Answer from the drawing. Dimensions are ordinates in mm from the lowest x, y and z of the part. Coordinates: 2 decimals unless noted, no trailing zeros. Write each loop counter-clockwise with the first axis right and the second up, starting at its lowest first coordinate (ties: lowest second). Pieces come first, ordered by that corner, then holes. Notation, with made-up numbers: (62.25, 21) - (102.25, 21) arc R22 cw to (102.25, 31) - close; hole circle Ø3 at (-13, -35.75). An arc over 180 degrees is marked (long way). Use a Markdown table: item, result.
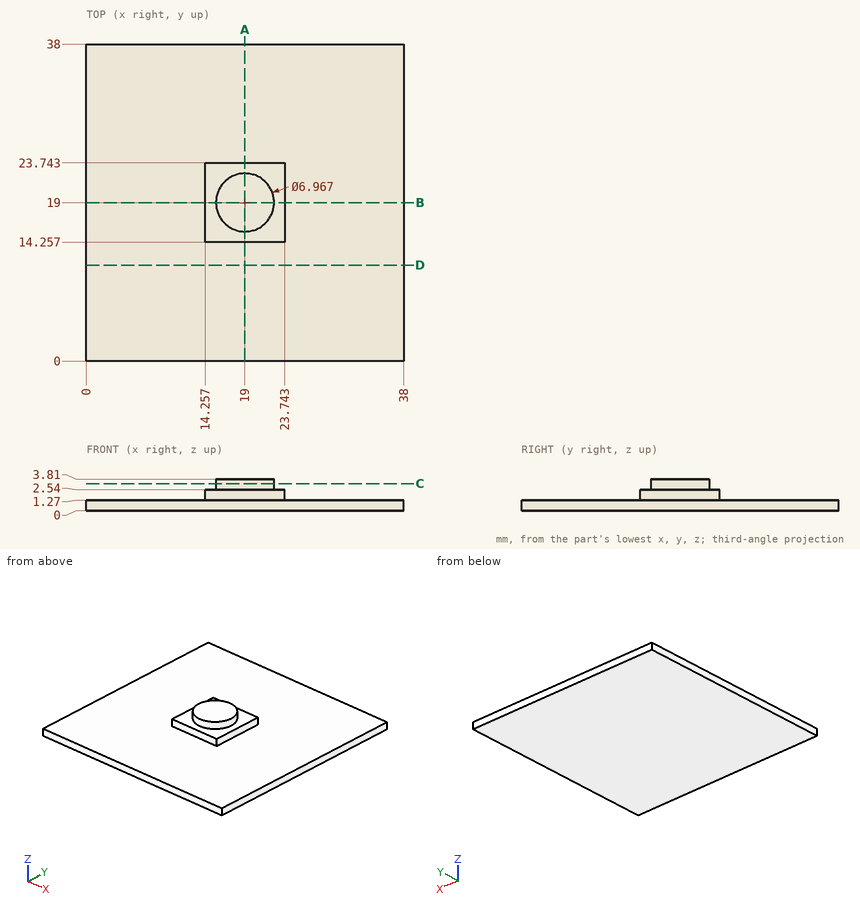
(1) A cutting plane is placed at A-A, the plane x = 19. Write down the section's boundary in (y, z).
Report:
| item | result |
|---|---|
| outline | (0, 0) - (38, 0) - (38, 1.27) - (23.74, 1.27) - (23.74, 2.54) - (22.48, 2.54) - (22.48, 3.81) - (15.52, 3.81) - (15.52, 2.54) - (14.26, 2.54) - (14.26, 1.27) - (0, 1.27) - close |
(2) Straight lines are drawn through the part: L1, parallel to Z at x = 16.5, y = 30; L2, parallel to Y at x = 22, z = 3.45; L3, parallel to Y at x = 18.5, z = 3. For each, find the intervals that lie inside material, in ascending order.
Report:
| item | result |
|---|---|
| L1 | z = 0 to 1.27 |
| L2 | y = 17.23 to 20.77 |
| L3 | y = 15.55 to 22.45 |
(3) A cutting plane is placed at D-D, the plane y = 11.5. Write down the section's boundary in (x, z).
Report:
| item | result |
|---|---|
| outline | (0, 0) - (38, 0) - (38, 1.27) - (0, 1.27) - close |
(4) A cutting plane is placed at C-C, the plane z = 3.25. Write down the section's boundary in (x, y), and give its area (3 significant figures).
Report:
| item | result |
|---|---|
| outline | circle Ø6.97 at (19, 19) |
| area | 38.1 mm² |
(5) Each of these flat-tipped pins is pushed along its axis until it touches: P1, Ø1, axis at x = 18.5, z = 2, coming from the -Y side; P2, Ø1, axis at x = 27.5, y = 32.5, coming from the +Z side; P3, Ø1.4, axis at x = 19, z = 2, coming from the +Y side. Where does it stop, or does it pass through?
Report:
| item | result |
|---|---|
| P1 | stops at y = 14.26 |
| P2 | stops at z = 1.27 |
| P3 | stops at y = 23.74 |
